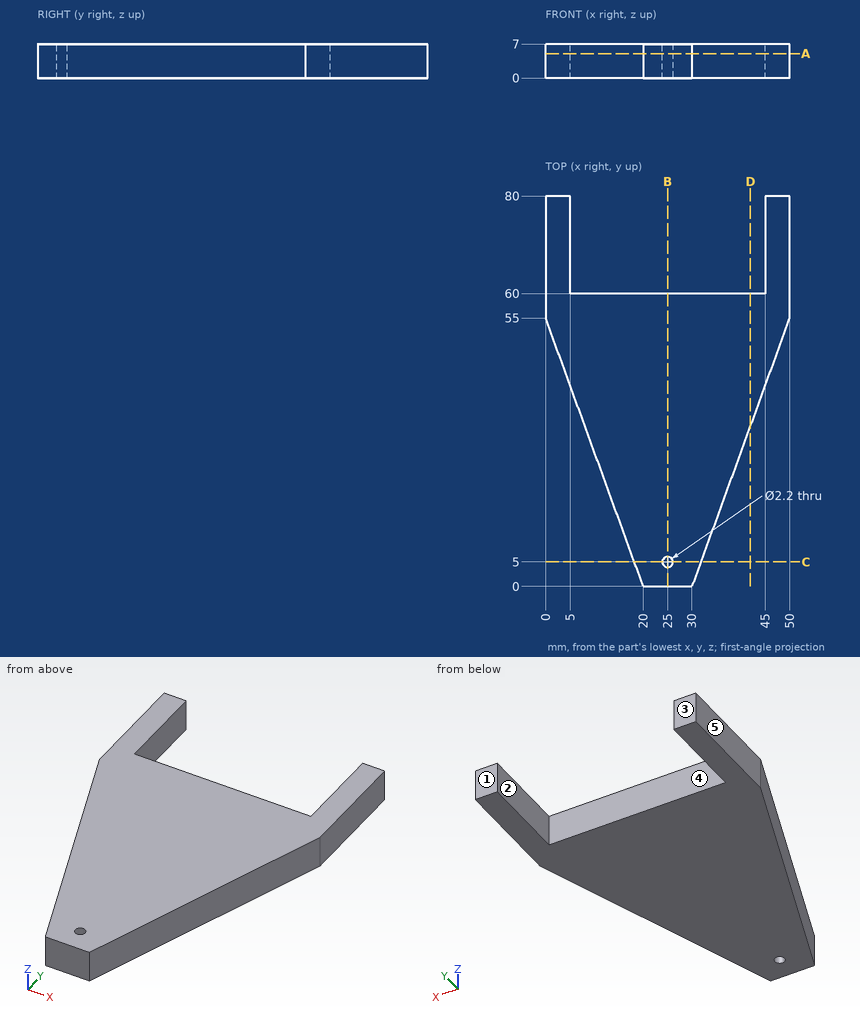
Verification items for this drawing (mm, ordinates from the low corner). A direction names the side the tool comes from. Give positions to 0.01 mm unless a question says otherwise; leave off trailing zeros. Loops run counter-clockwise (first coordinate to the right, second up) from the corner with the lowest first, then second, coordinate; pieces in that order, holes last. Notation, with made-up numbers: M 28.25,25.25 L 68.25,25.25 A19 cw 68.25,47.25 Z; hole C 21.25,31.5 d2. An arc over 180 degrees is marked long. Answer as a JSON object with one key per item and string values. Group by question number.
Q1. Release check for a two-part mould opening along X. For the marked faces 3, 4 and 5 record: released by +X, released by -X, zero draft, split by the parting line, or undercut.
Q2. Cross-section at B-B on x = 25. Record the cut outline in (y, z), then the cut area to 3 significant figures.
Q3. Material ranges on line 1 along Y through (x, z) = (25, 4); line 2 along X through (y, z) = (5, 2.5); line 3 along X through (y, z) = (51.5, 3), recorded low to high. Write a range as [from, to].
Q4. Cross-section at C-C on y = 5. Record the cut outline in (x, z), then the cut area to 3 significant figures.
Q5. Go/stop test with flat-tipped pins: P1, Ø4, axis at y = 14, z = 3.5, coming from the -X side; P2, Ø4, axis at y = 9, z = 3.5, coming from the +X side; P3, Ø1.5, axis at x = 36.5, z = 2.5, coming from the +Y side. Record where each tip stops, or that it passes through.
Q6. Cross-section at A-A on z = 5. Record the cut outline in (x, y), then the cut area to 3 significant figures.
Q7. Access from +Z, -Z, +X, -X, +Y, -Y to the whole of each face (thin tool, end or side, straight path). Record for the marked faces 1 and 2.
Q8. Cross-section at D-D on x = 42. Record the cut outline in (y, z), then the cut area to 3 significant figures.
Evaluation:
{
 "1": {"face 3": "zero draft", "face 4": "undercut", "face 5": "released by -X"},
 "2": {"outline": "M 0,0 L 3.9,0 L 3.9,7 L 0,7 Z; M 6.1,0 L 60,0 L 60,7 L 6.1,7 Z", "area": "405 mm2"},
 "3": {"line 1": "y = [0, 3.9], [6.1, 60]", "line 2": "x = [18.18, 23.9], [26.1, 31.82]", "line 3": "x = [1.27, 48.73]"},
 "4": {"outline": "M 18.18,0 L 23.9,0 L 23.9,7 L 18.18,7 Z; M 26.1,0 L 31.82,0 L 31.82,7 L 26.1,7 Z", "area": "80.1 mm2"},
 "5": {"P1": "stops at x = 14.18", "P2": "stops at x = 34", "P3": "stops at y = 60"},
 "6": {"outline": "M 0,55 L 20,0 L 30,0 L 50,55 L 50,80 L 45,80 L 45,60 L 5,60 L 5,80 L 0,80 Z; hole C 25,5 d2.2", "area": "2,100 mm2"},
 "7": {"face 1": "+Z, -Z, +X, -X, +Y", "face 2": "+Z, -Z, +Y"},
 "8": {"outline": "M 33,0 L 60,0 L 60,7 L 33,7 Z", "area": "189 mm2"}
}
